Check sheet for the modelled part. Datum: model origin and axes. Units: mm. Face numbers are marked on the shaded views. A direction names the side the tool comes from. Round coordinates to 2 decimals unless told otherwise and drop trailing zeros. Write each loop counter-clockwise with the first axis right and the second up, starting at its lowest first coordinate (ties: lowest second). Pieces come first, ordered by that corner, then holes. Notation, with made-up numbers: (-12.75, 75) -> (42.25, 75) arc R32 cw to (42.25, 103) -> close; hole circle Ø5 at (71, 57). An arc over 180 degrees is marked (long way). One line per item, written item: value. Start each with the question number.
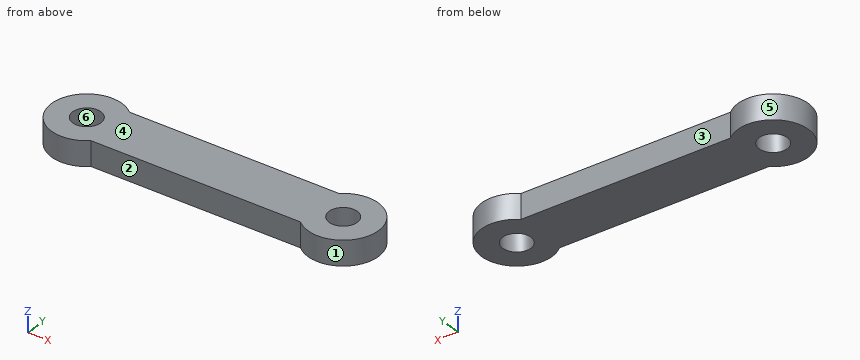
Autodesk Inventor part; units mm, degrees
ref_plane "YZ Plane" through (0, 0, 0) normal (1, 0, 0) x (0, 1, 0)
ref_plane "XZ Plane" through (0, 0, 0) normal (0, 1, 0) x (-1, 0, 0)
ref_plane "XY Plane" through (0, 0, 0) normal (0, 0, 1) x (1, 0, 0)
sketch "Sketch1" plane through (0, 0, 0) normal (0, 0, 1) x (1, 0, 0)
  arc A0 (3.3601, 3.81) -> (3.3601, -3.81) centre (0, 0) ccw
  circle A1 centre (0, 0) radius 2.032
  line L0 (3.3601, 3.81) -> (33.3683, 3.81)
  line L1 (3.3601, -3.81) -> (33.3683, -3.81)
  arc A2 (33.3683, -3.81) -> (33.3683, 3.81) centre (36.7284, 0) ccw
  circle A3 centre (36.7284, 0) radius 2.032
  dimension "d0" = 10.16
  dimension "d1" = 4.064
  dimension "d2" = 7.62
  dimension "d3" = 3.81
  dimension "d4" = 10.16
  dimension "d5" = 4.064
  dimension "d6" = 36.7284
extrude "Extrusion1" add sketch "Sketch1" along normal blind 3.556
equation "\"d5\" = d1"
properties part number "Arm 3"
1. Access from +Z, -Z, +X, -X, +Y, -Y to the whole of each face (thin tool, end or side, straight path). Record for the marked faces 1, 2 and 3.
2. Cross-section at C-C (z = 2.1). Record the cut outline in (x, y), plus the area to 3 significant figures.
3. Material ranges on probe 1 along Y at (x, z) = (0, 2.2); probe 2 along X at (y, z) = (1, 1.1); probe 3 along Y at (x, z) = (-1, 3.1), recorded low to high.
4. Release check for a two-part mould opening along X. For the marked faces 4, 5 and 6 record: +X half, -X half, draft (parallel to the pull), parting line (faces both ways), or undercut.
5. Cross-section at A-A (x = 0). Record the cut outline in (y, z), plus the area to 3 significant figures.
6. Cross-section at B-B (y = 0). Record the cut outline in (x, z), plus the area to 3 significant figures.
7. Cross-section at D-D (x = 28). Record the cut outline in (y, z), plus the area to 3 significant figures.
8. Depth check by flat-ended pin: pin 1 Ø1.1 at (x, z) = (19.5, 1.5) entering from +Y; pin 2 Ø1.5 at (x, z) = (32, 2.5) entering from -Y. Enter the tip coordinate at first touch or a pass-through.
Working result:
1. face 1: +Z, -Z
1. face 2: +Z, -Z, -Y
1. face 3: +Z, -Z, +Y
2. outline: (3.36, -3.81) -> (33.37, -3.81) arc R5.08 ccw (long way) to (33.37, 3.81) -> (3.36, 3.81) arc R5.08 ccw (long way) to start; hole circle Ø4.06 at (0, 0); hole circle Ø4.06 at (36.73, 0)
2. area: 347 mm^2
3. probe 1: y = -5.08 to -2.03, 2.03 to 5.08
3. probe 2: x = -4.98 to -1.77, 1.77 to 34.96, 38.5 to 41.71
3. probe 3: y = -4.98 to -1.77, 1.77 to 4.98
4. face 4: draft
4. face 5: undercut
4. face 6: undercut
5. outline: (-5.08, 0) -> (-2.03, 0) -> (-2.03, 3.56) -> (-5.08, 3.56) -> close; (2.03, 0) -> (5.08, 0) -> (5.08, 3.56) -> (2.03, 3.56) -> close
5. area: 21.7 mm^2
6. outline: (-5.08, 0) -> (-2.03, 0) -> (-2.03, 3.56) -> (-5.08, 3.56) -> close; (2.03, 0) -> (34.7, 0) -> (34.7, 3.56) -> (2.03, 3.56) -> close; (38.76, 0) -> (41.81, 0) -> (41.81, 3.56) -> (38.76, 3.56) -> close
6. area: 138 mm^2
7. outline: (-3.81, 0) -> (3.81, 0) -> (3.81, 3.56) -> (-3.81, 3.56) -> close
7. area: 27.1 mm^2
8. pin 1: stops at y = 3.81
8. pin 2: stops at y = -3.81
